from build123d import *

# Parameters (mm, degrees)
SKETCH_1_W          = 20.2
SKETCH_1_H          = 1.5
EXTRUDE_1_DEPTH     = 20
SKETCH_2_W          = 13
SKETCH_2_H          = 6
EXTRUDE_2_DEPTH     = 20
SKETCH_3_R          = 1
CUT_EXTRUDE_1_DEPTH = 2.5


with BuildPart() as part:
    # 草图1 → 凸台-拉伸1 (new body)
    with BuildSketch(Plane.XY):
        with Locations((-6.159701493, 0.302238806)):
            Rectangle(SKETCH_1_W, SKETCH_1_H)
    extrude(amount=-EXTRUDE_1_DEPTH)

    # 草图2 → 凸台-拉伸2 (add)
    with BuildSketch(Plane.XY):
        with Locations((-6.159701493, -3.447761194)):
            Rectangle(SKETCH_2_W, SKETCH_2_H)
    extrude(amount=-EXTRUDE_2_DEPTH)

    # 草图3 → 切除-拉伸1 (cut, through all)
    with BuildSketch(Plane(origin=(0, -0.447761194, 0), x_dir=(-1, 0, 0), z_dir=(0, -1, 0))):
        with Locations((-1.440298507, 17.5)):
            Circle(SKETCH_3_R)
        with Locations((13.759701493, 17.5)):
            Circle(SKETCH_3_R)
    extrude(amount=-CUT_EXTRUDE_1_DEPTH, mode=Mode.SUBTRACT)


solid = part.part
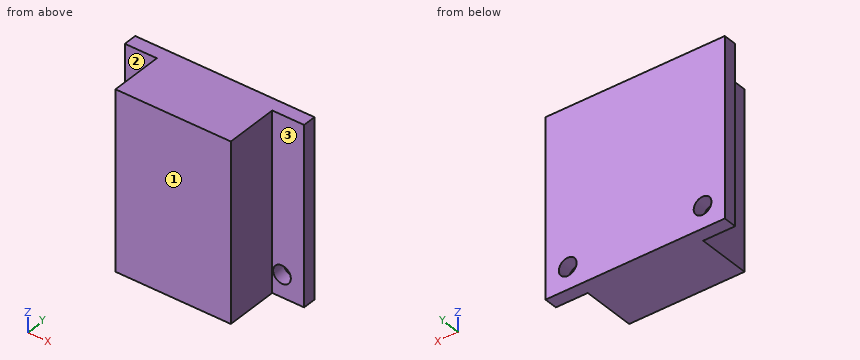
Here's how the part is built. I have some questions about the finished solid (model axes, mm). Face numbers are marked on the shaded views. A direction names the side the tool comes from. Give positions to 0.01 mm unless a question says otherwise; leave off trailing zeros. Order: outer loops, then holes, each group sorted by start corner. A loop starts at its lowest first (then second) coordinate and runs counter-clockwise, first axis right, second up. Notation, with made-up numbers: M -27.5,12 L 10.5,12 A21 cw 10.5,44 Z; hole C 19.5,64.5 d8. An arc over 180 degrees is marked long. Answer as a JSON object with one key per item and string values. Group by question number.
1) Please list where these lines run through material, in increasing order: L1, parallel to X at y = 0.7, z = -17.5; L2, parallel to X at y = -1.5, z = -12.5; L3, parallel to Y at x = -12.75, z = -18.25. Write a range as [from, to].
2) I'm going to push flat-ended pins straight in: pin 1 Ø4 at (x, z) = (2, -11) entering from -Y; pin 2 Ø1.8 at (y, z) = (-4.5, -10.5) entering from +X; pin 3 Ø3 at (y, z) = (-4, -12.5) entering from -X. Where does each tip first touch, or does it pass through?
3) Suppose I cut it at D-D, the plane y = -1. Write out the boundary of the cut face in (x, z), plus the area to 3 significant figures.
4) Suppose I cut it at A-A, the plane z = -17.5. Write out the boundary of the cut face in (x, y).
5) On a 3-axis mill with a long thin cutter (end or side, diameter ignored), from which of +Z, -Z, +X, -X, +Y, -Y can I reach the whole of each face in a straight line? I mean the marked faces 1, 2 and 3. Say none if no direction works.
6) Suppose I cut it at C-C, the plane x = -13.5. Write out the boundary of the cut face in (y, z), plus the area to 3 significant figures.
7) Suppose I cut it at B-B, the plane y = 0.75. Write out the boundary of the cut face in (x, z).
Results found:
{
 "1": {"L1": "[-16.26, -14.76], [-12.76, 0.44], [2.44, 3.94]", "L2": "[-12.66, 0.34]", "L3": "[-0.45, 1.05]"},
 "2": {"pin 1": "y = -6.45", "pin 2": "x = 0.34", "pin 3": "x = -12.66"},
 "3": {"outline": "M -12.66,-20 L 0.34,-20 L 0.34,0 L -12.66,0 Z", "area": "260 mm²"},
 "4": {"outline": "M -16.26,-0.45 L -14.76,-0.45 L -14.76,1.05 L -16.26,1.05 Z; M -12.76,-0.45 L -12.66,-0.45 L -12.66,-6.45 L 0.34,-6.45 L 0.34,-0.45 L 0.44,-0.45 L 0.44,1.05 L -12.76,1.05 Z; M 2.44,-0.45 L 3.94,-0.45 L 3.94,1.05 L 2.44,1.05 Z"},
 "5": {"face 1": "+Z, -Z, +X, -X, -Y", "face 2": "+Z, -Z, -X, -Y", "face 3": "+Z, -Z, +X, -Y"},
 "6": {"outline": "M -0.45,-20 L 1.05,-20 L 1.05,-18.47 L -0.45,-18.47 Z; M -0.45,-16.53 L 1.05,-16.53 L 1.05,0 L -0.45,0 Z", "area": "27.1 mm²"},
 "7": {"outline": "M -16.26,-20 L 3.94,-20 L 3.94,0 L -16.26,0 Z; hole C -13.76,-17.5 d2; hole C 1.44,-17.5 d2"}
}
